Answer from the drawing. Dimensions are ordinates in mm from the lowest x, y and z of the part. Coordinates: 2 decimals unless noted, no trailing zeros. Write each loop counter-clockwise with the first axis right and the second up, starting at its lowest first coordinate (ties: lowest second). Pieces come first, ordered by that corner, then holes. Notation, with made-up numbers: (62.25, 38.5) - (71.25, 38.5) arc R7 cw to (71.25, 43.5) - close; hole circle Ø4 at (50, 73). An arc over 180 degrees is marked (long way). Use one line per item in the form item = value. Start each with the question number.
Item 1: A cutting plane is placed at A-A (x = 23.4). Write down the section's boundary in (y, z), then the cut area to 3 significant figures.
Item 2: A cutting plane is placed at D-D (x = 59). Write down the section's boundary in (y, z), then the cut area to 3 significant figures.
Item 3: A cutting plane is placed at C-C (z = 1.5). Write down the section's boundary in (x, y), then the cut area to 3 significant figures.
Item 4: Consider probe 1 along X at (y, z) = (5.5, 1.55); probe 2 along Y at (x, z) = (23.4, 0.5); probe 3 along X at (y, z) = (2.75, 0.5). Determine where each line is inside the solid, lowest interval first.
Item 5: A cutting plane is placed at B-B (y = 5). Write down the section's boundary in (x, z), then the cut area to 4 significant figures.
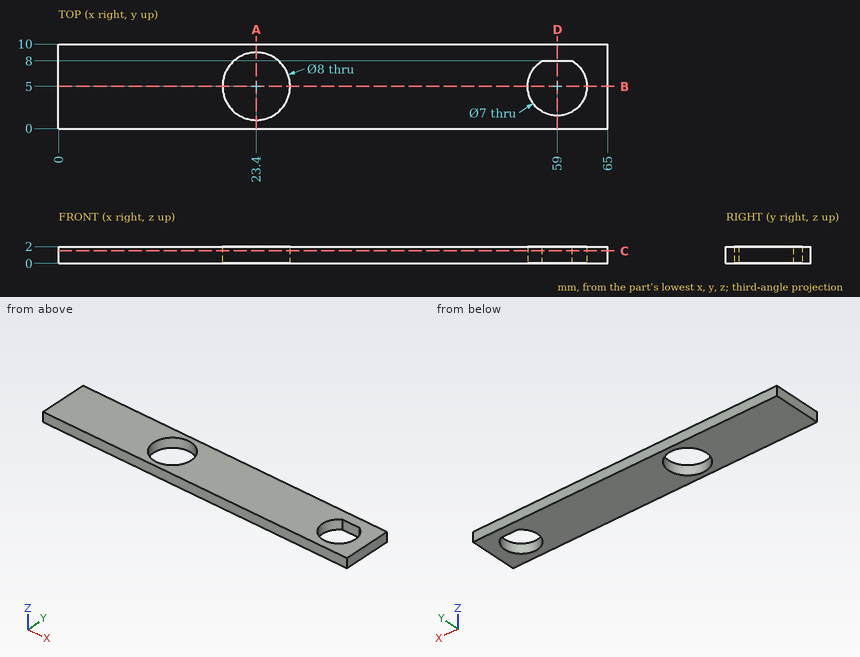
Answer:
q1.outline = (0, 0) - (1, 0) - (1, 2) - (0, 2) - close; (9, 0) - (10, 0) - (10, 2) - (9, 2) - close
q1.area = 4.00 mm²
q2.outline = (0, 0) - (1.5, 0) - (1.5, 2) - (0, 2) - close; (8, 0) - (10, 0) - (10, 2) - (8, 2) - close
q2.area = 7.00 mm²
q3.outline = (0, 0) - (65, 0) - (65, 10) - (0, 10) - close; hole circle Ø8 at (23.4, 5); hole (57.2, 8) arc R3.5 ccw (long way) to (60.8, 8) - close
q3.area = 562 mm²
q4.probe_1 = 0 to 19.43, 27.37 to 55.54, 62.46 to 65
q4.probe_2 = 0 to 1, 9 to 10
q4.probe_3 = 0 to 20.09, 26.71 to 56.32, 61.68 to 65
q5.outline = (0, 0) - (19.4, 0) - (19.4, 2) - (0, 2) - close; (27.4, 0) - (55.5, 0) - (55.5, 2) - (27.4, 2) - close; (62.5, 0) - (65, 0) - (65, 2) - (62.5, 2) - close
q5.area = 100.0 mm²
